Could you check a few things on this drawing? It's one solid part, dimensions in mm from its lowest x, y, z. A direction names the side the tool comes from. Round coordinates to 2 decimals unless told otherwise and drop trailing zeros. Loops run counter-clockwise (first coordinate to the right, second up) from the corner with the lowest first, then second, coordinate; pieces in that order, holes last. Notation, with made-up numbers: M 64,-7.75 L 103,-7.75 A10 ccw 103,9.25 Z; hole C 39,-4 d3. An arc over 180 degrees is marked long. Write each question's results on one line, items separated by ' | '. Start each with the question number.
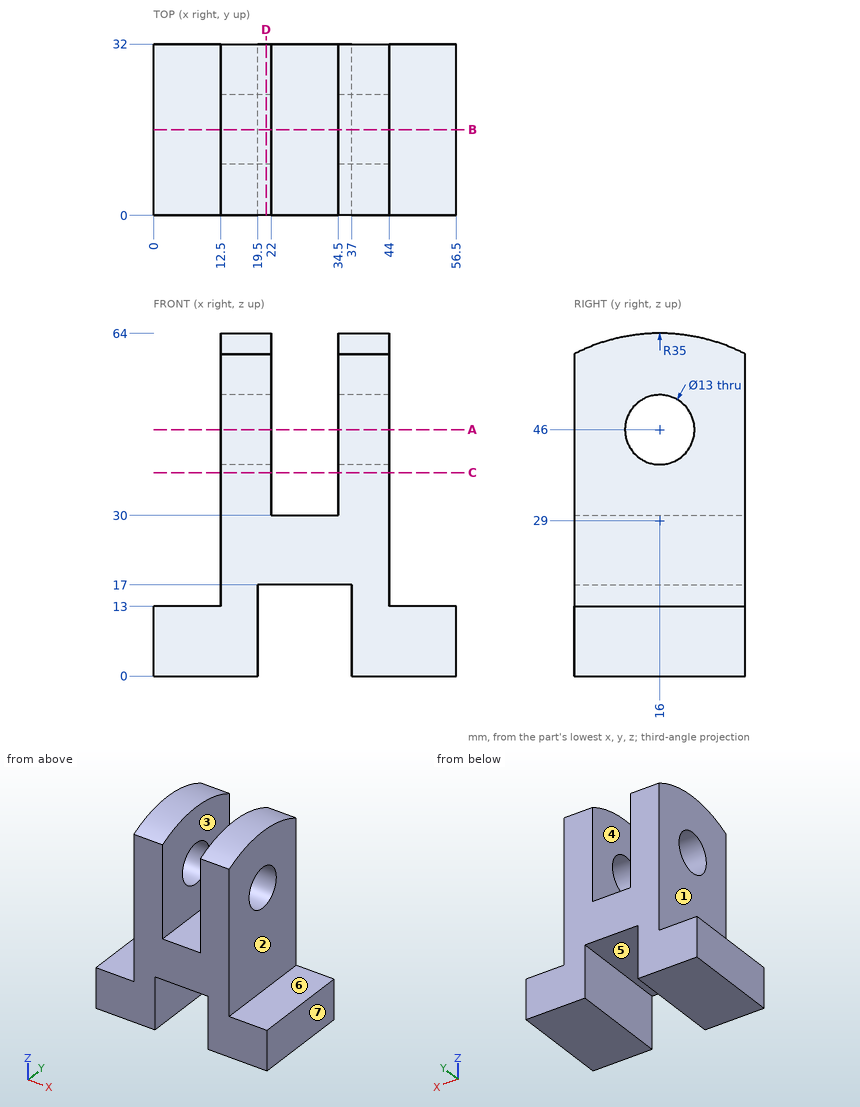
1. I want a section at C-C on z = 38. List the corners of the cut face in (x, y) for me.
2. I want a section at D-D on x = 21. List the corners of the cut face in (y, z) for me, plus the area to 3 significant figures.
3. I want a section at B-B on y = 16. List the corners of the cut face in (x, z) for me, plus the area to 3 significant figures.
4. I need wall thicknesses on line 1 along X through (y, z) = (4, 6.5); line 2 along X through (y, z) = (7, 35); line 3 along Z through (x, y) = (47, 4). Which ranges of each line are inside material? Lowest first, please.
5. I want a section at A-A on z = 46. List the corners of the cut face in (x, y) for me.
6. If we mould it in two halves opening along X, with no side actions, what happens to the marked faces 4, 5, 6 and 7? For each: released by +X, released by -X, zero draft, split by the parting line, or undercut.
7. Which directions (+Z, -Z, +X, -X, +Y, -Y) give clear straight access to the entire face, cutting with the end or side of a thin tool? Please do the marked faces 1, 2 and 3.
8. For pin 1 (10 mm diameter, centred on x = 26, y = 22.5, fed in from +Z); pin 2 (16 mm diameter, centred on y = 15, z = 48.5, fed in from +X); pin 3 (9.5 mm diameter, centred on y = 17.5, z = 47, fed in from -X); pin 4 (10 mm diameter, centred on x = 5.5, z = 50, fed in from -Y), each with a flat end and sliding along its axis, tell me the tip position at first contact or that it passes through.
Outcome:
1) outline: M 12.5,0 L 22,0 L 22,32 L 12.5,32 Z; M 34.5,0 L 44,0 L 44,32 L 34.5,32 Z
2) outline: M 0,17 L 32,17 L 32,60.13 A35 ccw 0,60.13 Z; hole C 16,46 d13 | area: 1,330 mm2
3) outline: M 0,0 L 19.5,0 L 19.5,17 L 37,17 L 37,0 L 56.5,0 L 56.5,13 L 44,13 L 44,39.5 L 34.5,39.5 L 34.5,30 L 22,30 L 22,39.5 L 12.5,39.5 L 12.5,13 L 0,13 Z; M 12.5,52.5 L 22,52.5 L 22,64 L 12.5,64 Z; M 34.5,52.5 L 44,52.5 L 44,64 L 34.5,64 Z | area: 1,370 mm2
4) line 1: 0 to 19.5, 37 to 56.5 | line 2: 12.5 to 22, 34.5 to 44 | line 3: 0 to 13
5) outline: M 12.5,0 L 22,0 L 22,9.5 L 12.5,9.5 Z; M 12.5,22.5 L 22,22.5 L 22,32 L 12.5,32 Z; M 34.5,0 L 44,0 L 44,9.5 L 34.5,9.5 Z; M 34.5,22.5 L 44,22.5 L 44,32 L 34.5,32 Z
6) face 4: undercut | face 5: undercut | face 6: zero draft | face 7: released by +X
7) face 1: +Z, -X, +Y, -Y | face 2: +Z, +X, +Y, -Y | face 3: +Z, +Y, -Y
8) pin 1: z = 63.82 | pin 2: x = 44 | pin 3: x = 12.5 | pin 4: through
